Study the drawing (mm; zero at the part's minimum x, y, z) and answer. A direction names the side the tool comes from. Round coordinates to 2 decimals unless told otherwise and drop trailing zeros. Write each loop counter-clockwise with the first axis right and the second up, starting at its lowest first coordinate (ties: lowest second). Pieces come first, ordered by that corner, then holes. Notation, with made-up numbers: (5.5, -2) - (13.5, -2) arc R28 ccw to (13.5, 34) - close; hole circle Ø1 at (17.25, 45). An arc over 180 degrees is marked (long way). Return JSON: item names as keys, results as strings. Group by question number.
(1) Section A-A, the plane x = 20 is taken. Write down the section's boundary in (y, z).
(2) Section D-D, the plane y = 5 is taken. Write down the section's boundary in (x, z), then the cut area to 3 significant figures.
(3) Section C-C, the plane z = 11.5 is taken. Write down the section's boundary in (x, y), then the cut area to 3 significant figures.
(4) Find the intervals of material crossed by line 1 along Y through (x, z) = (20, 17.25); line 2 along Z through (x, y) = (26, 3.5); line 3 along X through (y, z) = (9, 6.25), in increasing order. Write a range as [from, to].
(5) Which of the six approach directions +Z, -Z, +X, -X, +Y, -Y give full straight-line access (tool end or side, diameter ignored) to the marked faces 1, 2 and 3?
(6) Section B-B, the plane y = 20 is taken. Write down the section's boundary in (x, z).
(7) Each of these flat-tipped pins is pushed along its axis until it touches: pin 1 (3 mm diameter, centred on x = 16, z = 16, fed in from +Y); pin 2 (3 mm diameter, centred on x = 33, z = 16, fed in from -Y); pin 3 (8.5 mm diameter, centred on y = 26.5, z = 4.5, fed in from -X); pin 4 (23.5 mm diameter, centred on x = 20, y = 20, fed in from +Z) (3 decimals). Where does it stop, or does it pass through?
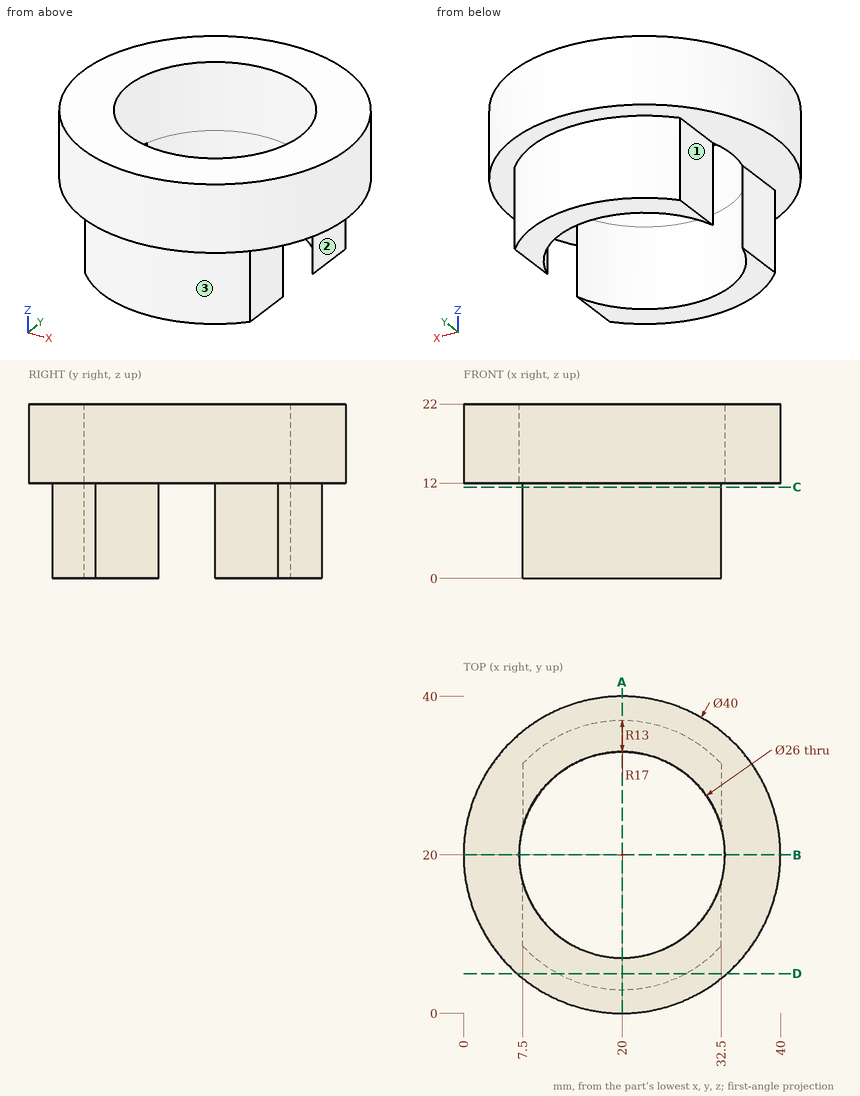
Working result:
{
 "1": {"outline": "(0, 12) - (3, 12) - (3, 0) - (7, 0) - (7, 22) - (0, 22) - close; (33, 0) - (37, 0) - (37, 12) - (40, 12) - (40, 22) - (33, 22) - close"},
 "2": {"outline": "(6.77, 12) - (12, 12) - (12, 0) - (28, 0) - (28, 12) - (33.23, 12) - (33.23, 22) - (6.77, 22) - close", "area": "457 mm^2"},
 "3": {"outline": "(7.5, 8.48) arc R17 ccw to (32.5, 8.48) - (32.5, 16.43) arc R13 cw to (7.5, 16.43) - close; (7.5, 23.57) arc R13 cw to (32.5, 23.57) - (32.5, 31.52) arc R17 ccw to (7.5, 31.52) - close", "area": "239 mm^2"},
 "4": {"line 1": "y = [0, 7], [33, 40]", "line 2": "z = [12, 22]", "line 3": "x = [7.5, 13.07], [26.93, 32.5]"},
 "5": {"face 1": "-Z, -X, +Y, -Y", "face 2": "-Z, +X, +Y, -Y", "face 3": "-Z, -Y"},
 "6": {"outline": "(0, 12) - (7, 12) - (7, 22) - (0, 22) - close; (33, 12) - (40, 12) - (40, 22) - (33, 22) - close"},
 "7": {"pin 1": "stops at y = 39.84", "pin 2": "stops at y = 3.64", "pin 3": "stops at x = 7.5", "pin 4": "passes through"}
}
